Design review of the part built by this model. Coordinates are the model's own, in mm. Coordinates: 2 decimals unless noted, no trailing zeros. Write each loop counter-clockwise with the first axis right and the second up, starting at its lowest first coordinate (ties: lowest second). Pieces come first, ordered by that corner, then holes.
Q1. Add section C-C, the plane x = 28. Give the boundary of the cut face in (y, z).
Q2. To check wall thickness, follow probe 1 along Y at (x, z) = (-50, 2.5); probe 2 along X at (y, z) = (-18, 5); probe 3 along Y at (x, z) = (0, 1.5). State the ranges of each line that lie inside material, in increasing order.
Q3. Add section D-D, the plane z = 1. Give the number of separate pieces and of enclosed holes in the cut face, plus the area to 3 significant figures.
Q4. Add section A-A, the plane y = 35. Give the boundary of the cut face in (x, z), plus the area to 3 significant figures.
Q5. Add section B-B, the plane x = -50. Give the boundary of the cut face in (y, z).
Q6. Clearance check with flat-ended pins moving along their axes: pin 1 Ø5.5 at (x, y) = (50, -40) entering from -Z; pin 2 Ø12 at (x, y) = (-0.5, 11) entering from -Z. State where each tip first meets the part, or that it passes through.
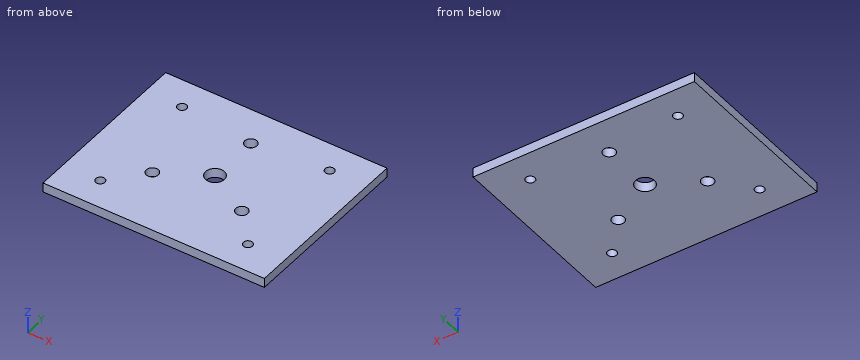
from build123d import *

# Parameters (mm, degrees)
CROQUIS1_W              = 150
CROQUIS1_H              = 120
CROQUIS1_R              = 4.1
CROQUIS1_R_2            = 3.1
CROQUIS1_R_3            = 6.35
SALIENTE_EXTRUIR1_DEPTH = 6.35


with BuildPart() as part:
    # Croquis1 → Saliente-Extruir1 (new body)
    with BuildSketch(Plane.XY):
        Rectangle(CROQUIS1_W, CROQUIS1_H)
        with Locations((0, 35)):
            Circle(CROQUIS1_R, mode=Mode.SUBTRACT)
        with Locations((-50, -40)):
            Circle(CROQUIS1_R_2, mode=Mode.SUBTRACT)
        with Locations((30.310889132, -17.5)):
            Circle(CROQUIS1_R, mode=Mode.SUBTRACT)
        with Locations((-30.310889132, -17.5)):
            Circle(CROQUIS1_R, mode=Mode.SUBTRACT)
        with Locations((50, -40)):
            Circle(CROQUIS1_R_2, mode=Mode.SUBTRACT)
        with Locations((50, 40)):
            Circle(CROQUIS1_R_2, mode=Mode.SUBTRACT)
        with Locations((-50, 40)):
            Circle(CROQUIS1_R_2, mode=Mode.SUBTRACT)
        Circle(CROQUIS1_R_3, mode=Mode.SUBTRACT)
    extrude(amount=SALIENTE_EXTRUIR1_DEPTH)


solid = part.part
Here are the results:
1. outline: (-60, 0) - (-20.89, 0) - (-20.89, 6.35) - (-60, 6.35) - close; (-14.11, 0) - (60, 0) - (60, 6.35) - (-14.11, 6.35) - close
2. probe 1: y = -60 to -43.1, -36.9 to 36.9, 43.1 to 60
2. probe 2: x = -75 to -34.38, -26.24 to 26.24, 34.38 to 75
2. probe 3: y = -60 to -6.35, 6.35 to 30.9, 39.1 to 60
3. separate pieces: 1
3. enclosed holes: 8
3. area: 17,600 mm2
4. outline: (-75, 0) - (-4.1, 0) - (-4.1, 6.35) - (-75, 6.35) - close; (4.1, 0) - (75, 0) - (75, 6.35) - (4.1, 6.35) - close
4. area: 900 mm2
5. outline: (-60, 0) - (-43.1, 0) - (-43.1, 6.35) - (-60, 6.35) - close; (-36.9, 0) - (36.9, 0) - (36.9, 6.35) - (-36.9, 6.35) - close; (43.1, 0) - (60, 0) - (60, 6.35) - (43.1, 6.35) - close
6. pin 1: passes through
6. pin 2: stops at z = 0
